from build123d import *

# Parameters (mm, degrees)
SKETCH1_R           = 7.9375
BOSS_EXTRUDE1_DEPTH = 19.05
SKETCH2_R           = 4.7625
CUT_EXTRUDE1_DEPTH  = 12.7
CHAMFER1_SIZE       = 1.5875


with BuildPart() as part:
    # Sketch1 → Boss-Extrude1 (new body)
    with BuildSketch(Plane.XY):
        Circle(SKETCH1_R)
    extrude(amount=BOSS_EXTRUDE1_DEPTH)

    # Sketch2 → Cut-Extrude1 (cut)
    with BuildSketch(Plane.XY.offset(19.05)):
        Circle(SKETCH2_R)
    extrude(amount=-CUT_EXTRUDE1_DEPTH, mode=Mode.SUBTRACT)

    # Chamfer1
    chamfer1_edges = [part.edges().sort_by_distance(p)[0] for p in [
        (-7.9375, 0, 0),
        (-7.9375, 0, 19.05),
    ]]
    chamfer(chamfer1_edges, length=CHAMFER1_SIZE)


solid = part.part
Part model, mm, in its own coordinate system. A direction names the side the tool comes from. Give positions to 0.01 mm unless a question says otherwise; leave off trailing zeros. Loops run counter-clockwise (first coordinate to the right, second up) from the corner with the lowest first, then second, coordinate; pieces in that order, holes last.
(1) Band-saw the part on D-D (z = 5.75). Write the cut outline in (x, y) (1 decimal).
Return value:
outline: circle Ø15.9 at (0, 0)
(2) Band-saw the part on B-B (x = 0). Write the cut outline in (y, z).
Return value:
outline: (-7.94, 1.59) - (-6.35, 0) - (6.35, 0) - (7.94, 1.59) - (7.94, 17.46) - (6.35, 19.05) - (4.76, 19.05) - (4.76, 6.35) - (-4.76, 6.35) - (-4.76, 19.05) - (-6.35, 19.05) - (-7.94, 17.46) - close
(3) 3-axis set-ups, long thin cutter, end or side, ignore diameter. For faces 4 (the flat face through (0, 0, 6.35)), 5 (the flat face through (0, 0, 0)): which of +Z, -Z, +X, -X, +Y, -Y reach the whole face in a straight line?
Return value:
face 4: +Z
face 5: -Z, +X, -X, +Y, -Y
(4) Pin check, flat tips, straight feed: pin 1 (1.5 mm diameter, centred on x = -3.5, z = 6.5, fed in from -Y); pin 2 (1 mm diameter, centred on x = 4, z = 10.5, fed in from -Y); pin 3 (6 mm diameter, centred on y = -5, z = 7.5, fed in from -X). Stop position of each tip, or through.
Return value:
pin 1: stops at y = -7.45
pin 2: stops at y = -7.12
pin 3: stops at x = -7.68
(5) Drill centre lines: line 1 along Y through (x, z) = (0, 10.5); line 2 along Y through (x, z) = (-1, 15.5); line 3 along Z through (x, y) = (1.5, 3). Where is each one in solid material? Low to high.
Return value:
line 1: y = -7.94 to -4.76, 4.76 to 7.94
line 2: y = -7.87 to -4.66, 4.66 to 7.87
line 3: z = 0 to 6.35
(6) Pull direction X, two halves, no side cores. Call faces 1 (the flat face through (1, 5, 19.05)), 2 (the cylindrical face through (-1.72, -7.75, 9.41)), 3 (the cylindrical face through (-3.78, -2.9, 12.79)): pulls with the +X half, pulls with the -X half, needs draft (parallel to the pull), parting line crosses it, or undercut.
Return value:
face 1: needs draft
face 2: parting line crosses it
face 3: undercut
(7) Band-saw the part on A-A (z = 18). Write the cut outline in (x, y) (1 decimal), and give its area (3 significant figures).
Return value:
outline: circle Ø14.8 at (0, 0); hole circle Ø9.5 at (0, 0)
area: 101 mm2
